Autodesk Inventor part; units mm, degrees
ref_plane "YZ Plane" through (0, 0, 0) normal (1, 0, 0) x (0, 1, 0)
ref_plane "XZ Plane" through (0, 0, 0) normal (0, 1, 0) x (-1, 0, 0)
ref_plane "XY Plane" through (0, 0, 0) normal (0, 0, 1) x (1, 0, 0)
sketch "草圖1" plane through (0, 0, 0) normal (1, 0, 0) x (0, 1, 0)
  line L0 (-37.5, 37.5) -> (37.5, 37.5)
  line L1 (37.5, 37.5) -> (37.5, -37.5)
  line L2 (37.5, -37.5) -> (-37.5, -37.5)
  line L3 (-37.5, -37.5) -> (-37.5, 37.5)
  line L4 (-37.5, 37.5) -> (37.5, -37.5) construction
  line L5 (37.5, 37.5) -> (-37.5, -37.5) construction
  point P0 (0, 0)
  dimension "d0" = 75
  dimension "d1" = 75
extrude "擠出1" add sketch "草圖1" along normal blind 20
fillet "圓角1" radius 30 4 edges at (10, 37.5, 37.5) (10, -37.5, 37.5) (10, 37.5, -37.5) (10, -37.5, -37.5)
chamfer "倒角1" distance 10 angle 45 8 edges at (20, 0, 37.5) (20, -28.7132, 28.7132) (20, -37.5, 0) (20, -28.7132, -28.7132) (20, 0, -37.5) (20, 28.7132, -28.7132) (20, 37.5, 0) (20, 28.7132, 28.7132)
sketch "草圖2" plane through (20, 0, 0) normal (1, 0, 0) x (0, 0, -1)
  line L0 (0, 0) -> (0, 0)
  line L1 (0, 0) -> (0, 0)
  line L2 (0, 0) -> (0, 0)
  line L3 (0, 0) -> (0, 0)
  line L4 (0, 0) -> (0, 0) construction
  line L5 (0, 0) -> (0, 0) construction
  point P0 (0, 0)
  dimension "d8" = 0
  dimension "d9" = 0
hole "孔1" at (20, 0, 0) at (20, 0, 0) at (20, 0, 0) at (20, 0, 0) direction (-1, 0, 0) diameter 12 depth 10 tip angle 118
sketch "草圖3" plane through (0, 0, 0) normal (-1, 0, 0) x (0, 0, 1)
  arc A0 (-37.5, -7.5) -> (-7.5, -37.5) centre (-7.5, -7.5) ccw
  line L0 (-7.5, -37.5) -> (7.5, -37.5)
  arc A1 (7.5, -37.5) -> (37.5, -7.5) centre (7.5, -7.5) ccw
  line L1 (37.5, -7.5) -> (37.5, 7.5)
  arc A2 (37.5, 7.5) -> (7.5, 37.5) centre (7.5, 7.5) ccw
  line L2 (7.5, 37.5) -> (-7.5, 37.5)
  arc A3 (-7.5, 37.5) -> (-37.5, 7.5) centre (-7.5, 7.5) ccw
  line L3 (-37.5, 7.5) -> (-37.5, -7.5)
  line L4 (12.5, 12.5) -> (-12.5, 12.5)
  line L5 (-12.5, 12.5) -> (-12.5, -12.5)
  line L6 (-12.5, -12.5) -> (12.5, -12.5)
  line L7 (12.5, -12.5) -> (12.5, 12.5)
  line L8 (12.5, 12.5) -> (-12.5, -12.5) construction
  line L9 (-12.5, 12.5) -> (12.5, -12.5) construction
  point P0 (0, 0)
  dimension "d17" = 25
  dimension "d18" = 25
hole "孔2" at (0, -12.5, 12.5) at (0, -12.5, -12.5) at (0, 12.5, -12.5) at (0, 12.5, 12.5) direction (1, 0, 0) diameter 12 depth 10 tip angle 118
properties part number "exercise3-1-6"
The listing builds one solid part. Answer for the finished solid, in the listing's coordinates (mm). A direction names the side the tool comes from. Coordinates: 2 decimals unless noted, no trailing zeros. Loops run counter-clockwise (first coordinate to the right, second up) from the corner with the lowest first, then second, coordinate; pieces in that order, holes last. Notation, with made-up numbers: M 60.5,9.25 L 101.5,9.25 A14 cw 101.5,32.25 Z; hole C 39.5,85.25 d8. An arc over 180 degrees is marked long. Answer as CSV lines item,"result". Start each with the question number.
(1) The part is cut by section C-C (x = 8.75). Give the vertices of the cut face in (y, z).
(2) Find the intervals of material crossed by L1, parallel to Y at x = 3.5, z = 12.5; L2, parallel to Z at x = 3, y = 16, in increasing order. Write a range as [from, to].
(3) The mould has two halves that part along Z. Classify faces 3 (the flat face through (15.1, 32.4, -0.1)), 4 (the cylindrical face through (5.07, -7.177, -9.731)), 5 (the flat face through (15.1, -0.1, -32.4)): pulls with the +Z half, pulls with the -Z half, needs draft (parallel to the pull), parting line crosses it, or undercut.
(4) Given pin 1 (5 mm diameter, centred on x = 3.5, y = 28.5, fed in from -Z); pin 2 (11 mm diameter, centred on y = -12.5, z = 12.5, fed in from -X); pin 3 (1 mm diameter, centred on y = -25.5, z = 26, fed in from +X), each flat-ended and moving along its own axis, determine where each tip first touches the part or whether it passes through.
(5) The part is cut by section B-B (x = 18.25). Give the vertices of the cut face in (y, z).
(6) For faces 1 (the cylindrical face through (5.07, 7.441, -9.274)), 2 (the cylindrical face through (5.07, -28.945, -28.479)), determine the directions among +Z, -Z, +X, -X, +Y, -Y from which every point of the face is accessible in a straight line to the end or side of a thin tool.
(7) The part is cut by section A-A (x = 3.75). Give the vertices of the cut face in (y, z), and give its area (3 significant figures).
Determined:
1,outline,"M -37.5,-7.5 A30 ccw -7.5,-37.5 L 7.5,-37.5 A30 ccw 37.5,-7.5 L 37.5,7.5 A30 ccw 7.5,37.5 L -7.5,37.5 A30 ccw -37.5,7.5 Z; hole C -12.5,-12.5 d12; hole C -12.5,12.5 d12; hole C 0,0 d7.84; hole C 12.5,-12.5 d12; hole C 12.5,12.5 d12"
2,L1,"[-37.08, -18.5], [-6.5, 6.5], [18.5, 37.08]"
2,L2,"[-36.27, -17.37], [-7.63, 7.63], [17.37, 36.27]"
3,face 3,"needs draft"
3,face 4,"undercut"
3,face 5,"pulls with the -Z half"
4,pin 1,"z = -31.12"
4,pin 2,"x = 10.3"
4,pin 3,"x = 14.69"
5,outline,"M -29.25,-7.5 A21.75 ccw -7.5,-29.25 L 7.5,-29.25 A21.75 ccw 29.25,-7.5 L 29.25,7.5 A21.75 ccw 7.5,29.25 L -7.5,29.25 A21.75 ccw -29.25,7.5 Z; hole C 0,0 d12"
6,face 1,"-X"
6,face 2,"-Z, +X, -X, -Y"
7,outline,"M -37.5,-7.5 A30 ccw -7.5,-37.5 L 7.5,-37.5 A30 ccw 37.5,-7.5 L 37.5,7.5 A30 ccw 7.5,37.5 L -7.5,37.5 A30 ccw -37.5,7.5 Z; hole C -12.5,-12.5 d12; hole C -12.5,12.5 d12; hole C 12.5,-12.5 d12; hole C 12.5,12.5 d12"
7,area,"4,400 mm2"
